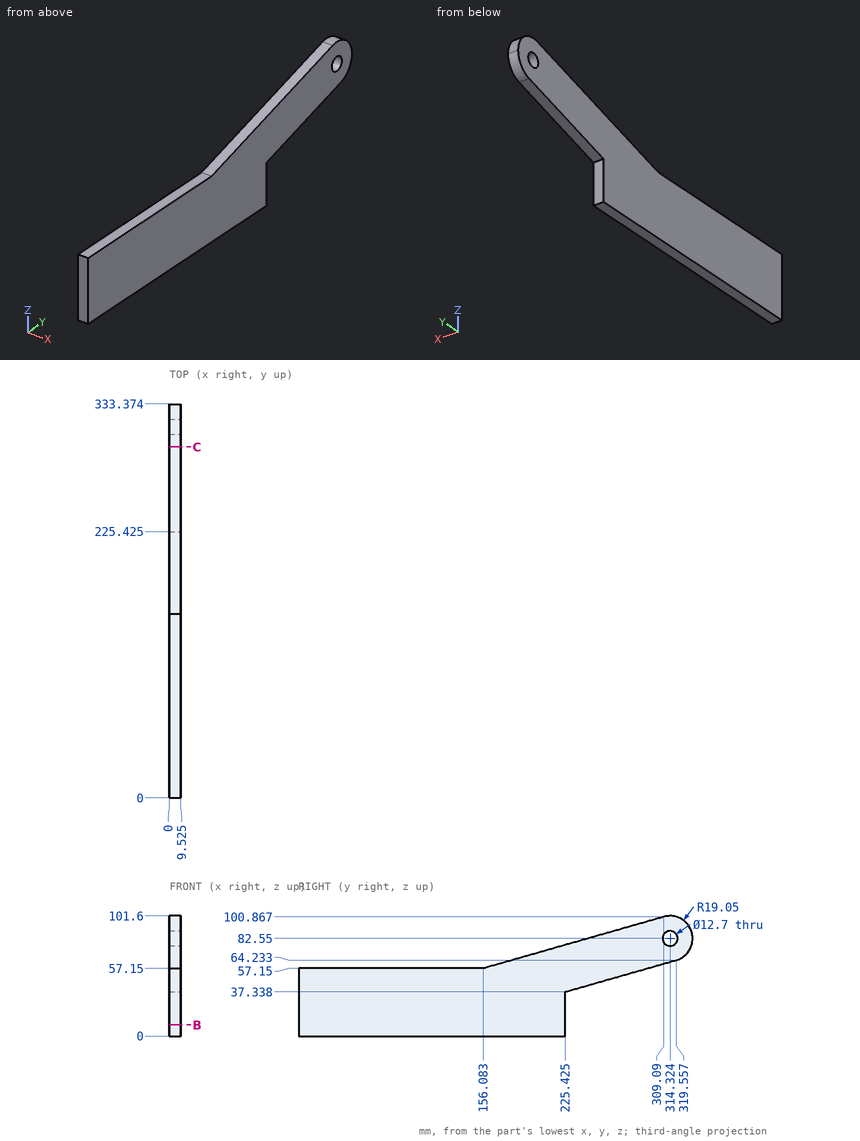
Here's the drawing with two shaded views (mm, measured from the low corner). I have some questions. Give positions to 0.01 mm unless a question says otherwise; leave off trailing zeros. Loops run counter-clockwise (first coordinate to the right, second up) from the corner with the lowest first, then second, coordinate; pieces in that order, holes last. Notation, with made-up numbers: M -37.5,23.25 L 13.5,23.25 A20 ccw 13.5,46.25 Z; hole C -40,39.5 d2. An arc over 180 degrees is marked long. One line per item, written item: value.
(1) Will these pins go through, and if not, where does the flat tip stop? pin 1 (1 mm diameter, centred on x = 8, y = 36, fed in from +Z); pin 2 (3 mm diameter, centred on x = 5, z = 16, fed in from +Y) (3 decimals); pin 3 (3 mm diameter, centred on x = 3.5, y = 238, fed in from +Z).
Returned:
pin 1: z = 57.15
pin 2: y = 225.425
pin 3: z = 80.98
(2) Suppose I cut it at C-C on y = 297. List the corners of the cut face in (x, z) for me (1 decimal).
Returned:
outline: M 0,57.8 L 9.5,57.8 L 9.5,97.4 L 0,97.4 Z
(3) I need wall thicknesses on line 1 (Z direction, x = 1.25, y = 147); line 2 (Y direction, x = 4, z = 19.5) (1 decimal); line 3 (Z direction, x = 1.5, y = 261). Which ranges of each line are inside material? Lowest first, please.
Returned:
line 1: 0 to 57.15
line 2: 0 to 225.4
line 3: 47.5 to 87.13
(4) Suppose I cut it at B-B on z = 9.5. List the corners of the cut face in (x, y) for me (1 decimal), plus the area to 3 significant figures.
Returned:
outline: M 0,0 L 9.5,0 L 9.5,225.4 L 0,225.4 Z
area: 2,150 mm^2
